Answer from the drawing. Dimensions are ordinates in mm from the lowest x, y and z of the part. A direction names the side the tool comes from. Round coordinates to 2 decimals unless told otherwise and drop trailing zeros. Write each loop counter-clockwise with the first axis right and the second up, starting at its lowest first coordinate (ties: lowest second). Pieces come first, ordered by that corner, then holes. Notation, with made-up numbers: (47, -5) - (63, -5) arc R17 cw to (63, 8) - close; hole circle Ø7 at (23.25, 48.25). An arc over 180 degrees is marked (long way). Answer in a Markdown table with one row per item.
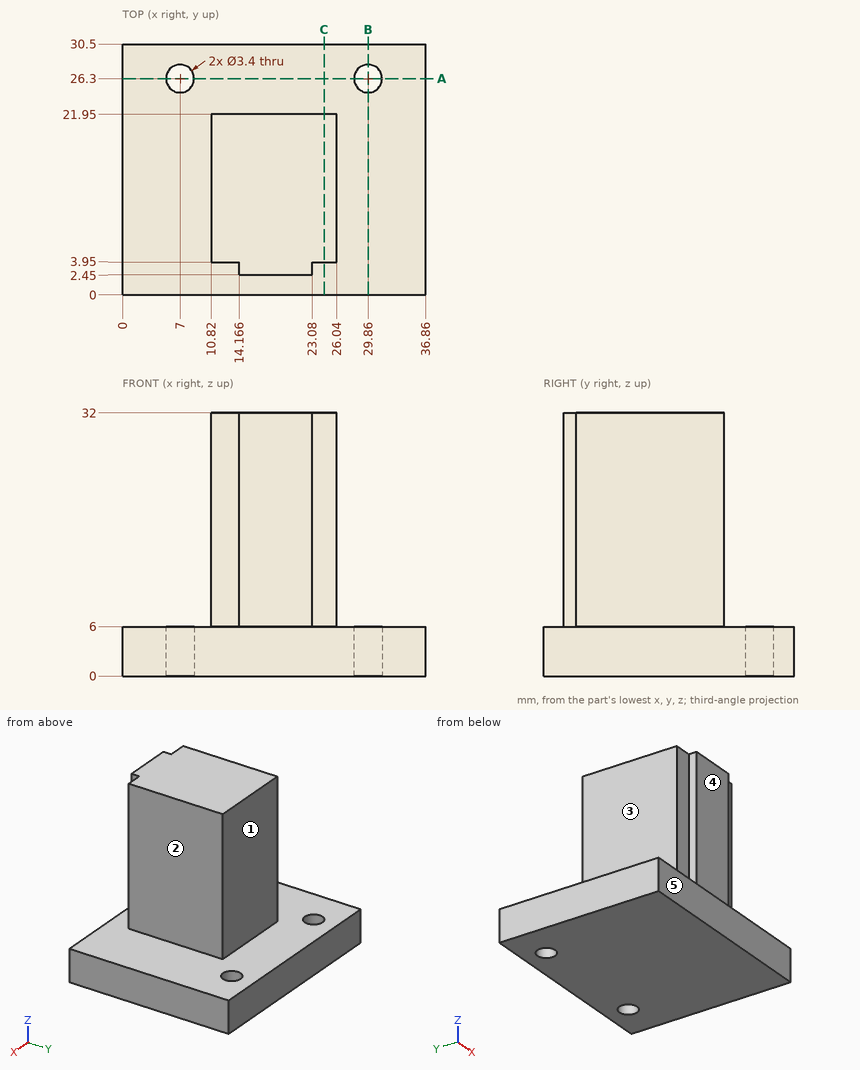
(1) Flat-ended cylindrical pins translate along their axes: pin 1 (12 mm diameter, centred on x = 16, z = 21, fed in from +Y); pin 2 (6 mm diameter, centred on y = 6.5, z = 17.5, fed in from -X); pin 3 (6 mm diameter, centred on y = 20.5, z = 14, fed in from +X); pin 4 (3 mm diameter, centred on x = 7, y = 26.3, fed in from -Z). Find the tip coordinate at first contact, or state that the pin passes through.
Checked values:
| item | result |
|---|---|
| pin 1 | stops at y = 21.95 |
| pin 2 | stops at x = 10.82 |
| pin 3 | stops at x = 26.04 |
| pin 4 | passes through |
(2) For the marked faces 1, 2, 3, 4 and 5, determine the directions among +Z, -Z, +X, -X, +Y, -Y from which every point of the face is accessible in a straight line to the end or side of a thin tool.
Checked values:
| item | result |
|---|---|
| face 1 | +Z, +X, -X, +Y |
| face 2 | +Z, +X, +Y, -Y |
| face 3 | +Z, -X, +Y, -Y |
| face 4 | +Z, +X, -X, -Y |
| face 5 | +Z, -Z, +X, -X, -Y |
(3) Section C-C (x = 24.5) is taken. Give the vertices of the cut face in (y, z), and give its area (3 significant figures).
Checked values:
| item | result |
|---|---|
| outline | (0, 0) - (30.5, 0) - (30.5, 6) - (21.95, 6) - (21.95, 32) - (3.95, 32) - (3.95, 6) - (0, 6) - close |
| area | 651 mm2 |
(4) Section B-B (x = 29.86) is taken. Give the vertices of the cut face in (y, z), and give its area (3 significant figures).
Checked values:
| item | result |
|---|---|
| outline | (0, 0) - (24.6, 0) - (24.6, 6) - (0, 6) - close; (28, 0) - (30.5, 0) - (30.5, 6) - (28, 6) - close |
| area | 163 mm2 |
(5) Section A-A (y = 26.3) is taken. Give the vertices of the cut face in (x, z).
Checked values:
| item | result |
|---|---|
| outline | (0, 0) - (5.3, 0) - (5.3, 6) - (0, 6) - close; (8.7, 0) - (28.16, 0) - (28.16, 6) - (8.7, 6) - close; (31.56, 0) - (36.86, 0) - (36.86, 6) - (31.56, 6) - close |
(6) Find the intervals of material crossed by line 1 (Y direction, x = 29.86, z = 4.6); line 2 (X direction, y = 26, z = 2); line 3 (X direction, y = 3, z = 16) (1 decimal), in increasing order.
Checked values:
| item | result |
|---|---|
| line 1 | y = 0 to 24.6, 28 to 30.5 |
| line 2 | x = 0 to 5.33, 8.67 to 28.19, 31.53 to 36.86 |
| line 3 | x = 14.2 to 23.1 |
